Geometry: final body of the model. Coordinates: model frame, mm. A direction names the side the tool comes from. Give positions to 0.01 mm unless a question says otherwise; leave off trailing zeros. Write each loop counter-clockwise with the first axis right and the second up, starting at its lowest first coordinate (ties: lowest second). Pieces come first, ordered by that corner, then holes. Notation, with made-up numbers: M 35,67.5 L 54,67.5 A29 ccw 54,97.5 Z; hole C 80,63 d3. An arc over 180 degrees is marked long. Answer as a JSON object with one key per item and string values.
from build123d import *

# Parameters (mm, degrees)
THICKEN1_START   = -2
THICKEN1_DEPTH   = 2
THICKEN1_2_DEPTH = 10


# Read off the part's stored shape, not the designer's step: Thicken1
with BuildPart() as part:
    # Thicken1 outline → Thicken1 (new body)
    with BuildSketch(Plane.XY.offset(THICKEN1_START)):
        with BuildLine():
            Line((-87, -44.9), (87, -44.9))
            ThreePointArc((87, -44.9), (88.767766953, -44.167766953), (89.5, -42.4))
            Line((89.5, -42.4), (89.5, 42.4))
            ThreePointArc((89.5, 42.4), (88.767766953, 44.167766953), (87, 44.9))
            Line((87, 44.9), (-87, 44.9))
            ThreePointArc((-87, 44.9), (-88.767766953, 44.167766953), (-89.5, 42.4))
            Line((-89.5, 42.4), (-89.5, -42.4))
            ThreePointArc((-89.5, -42.4), (-88.767766953, -44.167766953), (-87, -44.9))
        make_face()
    extrude(amount=THICKEN1_DEPTH)

    # Thicken1 2 outline → Thicken1 2 (add)
    with BuildSketch(Plane.XY):
        with BuildLine():
            Line((-87, -44.9), (87, -44.9))
            ThreePointArc((87, -44.9), (88.767766953, -44.167766953), (89.5, -42.4))
            Line((89.5, -42.4), (89.5, 42.4))
            ThreePointArc((89.5, 42.4), (88.767766953, 44.167766953), (87, 44.9))
            Line((87, 44.9), (-87, 44.9))
            ThreePointArc((-87, 44.9), (-88.767766953, 44.167766953), (-89.5, 42.4))
            Line((-89.5, 42.4), (-89.5, -42.4))
            ThreePointArc((-89.5, -42.4), (-88.767766953, -44.167766953), (-87, -44.9))
        make_face()
        with BuildLine():
            ThreePointArc((87.5, -42.4), (87.353553391, -42.753553391), (87, -42.9))
            Line((87, -42.9), (-87, -42.9))
            ThreePointArc((-87, -42.9), (-87.353553391, -42.753553391), (-87.5, -42.4))
            Line((-87.5, -42.4), (-87.5, 42.4))
            ThreePointArc((-87.5, 42.4), (-87.353553391, 42.753553391), (-87, 42.9))
            Line((-87, 42.9), (87, 42.9))
            ThreePointArc((87, 42.9), (87.353553391, 42.753553391), (87.5, 42.4))
            Line((87.5, 42.4), (87.5, -42.4))
        make_face(mode=Mode.SUBTRACT)
    extrude(amount=THICKEN1_2_DEPTH)


solid = part.part
1) Cut plane B-B on x = 38. Return loops of the section in (y, z), and give its area (3 significant figures).
Geometry check:
{"outline": "M -44.9,-2 L 44.9,-2 L 44.9,10 L 42.9,10 L 42.9,0 L -42.9,0 L -42.9,10 L -44.9,10 Z", "area": "220 mm2"}
2) Pull-direction query (X, two-part tool) for faces 1 (the flat face through (87.5, 1, 5)), 2 (the flat face through (-0.4, 43.4, 10)), 3 (the flat face through (-87.5, -1, 5)), 4 (the flat face through (89.5, -1, 4)); classes: pulls with the +X half, pulls with the -X half, needs draft (parallel to the pull), parting line crosses it, or undercut.
Geometry check:
{"face 1": "undercut", "face 2": "needs draft", "face 3": "undercut", "face 4": "pulls with the +X half"}
3) Contact query for a flat-ended pin moving along its axis: P1, Ø4, axis at x = 45, y = -1, coming from the +Z side. Output: stop coordinate, or through.
Geometry check:
{"P1": "stops at z = 0"}
4) Cut plane C-C on y = 20.5. Return loops of the section in (x, z).
Geometry check:
{"outline": "M -89.5,-2 L 89.5,-2 L 89.5,10 L 87.5,10 L 87.5,0 L -87.5,0 L -87.5,10 L -89.5,10 Z"}
5) Set-up query: faces 5 (the flat face through (1, -42.9, 5)), 6 (the flat face through (-1, 1, -2)). Return all of +Z, -Z, +X, -X, +Y, -Y with unobstructed straight access to the full face (end or side cutting, diameter ignored); none if empty.
Geometry check:
{"face 5": "+Z", "face 6": "-Z, +X, -X, +Y, -Y"}
6) Cut plane A-A on z = 7. Return loops of the section in (x, y).
Geometry check:
{"outline": "M -89.5,-42.4 A2.5 ccw -87,-44.9 L 87,-44.9 A2.5 ccw 89.5,-42.4 L 89.5,42.4 A2.5 ccw 87,44.9 L -87,44.9 A2.5 ccw -89.5,42.4 Z; hole M -87.5,-42.4 A0.5 ccw -87,-42.9 L 87,-42.9 A0.5 ccw 87.5,-42.4 L 87.5,42.4 A0.5 ccw 87,42.9 L -87,42.9 A0.5 ccw -87.5,42.4 Z"}
7) Line query: line 1 (Y direction, x = -69.5, z = 8.25); line 2 (X direction, y = -39.5, z = 7); line 3 (Z direction, x = -20, y = 39). Output: solid intervals per line, ascending. Write a range as from..to.
Geometry check:
{"line 1": "y = -44.9..-42.9, 42.9..44.9", "line 2": "x = -89.5..-87.5, 87.5..89.5", "line 3": "z = -2..0"}
